from build123d import *

# Parameters (mm, degrees)
F0_R     = 20
F1_DEPTH = 20
F2_R     = 10
F3_R     = 9
F4_DEPTH = 20
F5_R     = 2.5
F6_DEPTH = 20
F7_SIZE  = 1.5


with BuildPart() as f1:
    # F0 (on Top) → F1 (new body)
    with BuildSketch(Plane.XY):
        Circle(F0_R)
    extrude(amount=F1_DEPTH)

    # F2
    f2_edges = [f1.edges().sort_by_distance(p)[0] for p in [
        (-20, 0, 0),
    ]]
    fillet(f2_edges, radius=F2_R)

    # F3 (on face) → F4 (join)
    with BuildSketch(Plane.XY.offset(20)):
        Circle(F3_R)
    extrude(amount=F4_DEPTH)

    # F5 (on face) → F6 (cut)
    with BuildSketch(Plane.XY.offset(40)):
        Circle(F5_R)
    extrude(amount=-F6_DEPTH, mode=Mode.SUBTRACT)

    # F7
    f7_edges = [f1.edges().sort_by_distance(p)[0] for p in [
        (-20, 0, 20),
    ]]
    chamfer(f7_edges, length=F7_SIZE)


solid = f1.part
Could you check a few things on this model? Use its own coordinates, in mm. A direction names the side the tool comes from. Coordinates: 2 decimals unless noted, no trailing zeros. Order: outer loops, then holes, each group sorted by start corner. A loop starts at its lowest first (then second) coordinate and runs counter-clockwise, first axis right, second up. Notation, with made-up numbers: (12, -27.75) - (62, -27.75) arc R11 cw to (62, -8.75) - close; hole circle Ø6 at (61.25, 8.25). An arc over 180 degrees is marked (long way). Answer in a Markdown table with one row per item. Add a question column.
(1) Will these pins go through, and if not, where does the flat tip stop? pin 1 (2 mm diameter, centred on x = 0, y = 15.5, fed in from +Z); pin 2 (1 mm diameter, centred on y = 0.5, z = 33, fed in from -X); pin 3 (1.5 mm diameter, centred on x = -3.5, z = 32.5, fed in from +Y).
(2) If we section it at A-A, the plane z = 34: Please give me the cut outline in (x, y), then the cut area to 3 significant figures.
(3) I need wall thicknesses on L1, parallel to Y at x = 0, z = 33.25; L2, parallel to Y at x = 7, z = 24.5; L3, parallel to Y at x = -17, z = 5. Which ranges of each line are inside material? Lowest first, please.
(4) On a 3-axis mill with a long thin cutter (end or side, diameter ignored), from which of +Z, -Z, +X, -X, +Y, -Y can I reach the whole of each face in a straight line? I mean faces 4 (the face through (2, -2, 40)), 5 (the face through (-0.54, -2.44, 30.14)). Say none if no direction works.
(5) If we mould it in two halves opening along Y, with no side actions, what happens to faces 1 (the face through (3.9, 8.5, 20)), 2 (the face through (0, 0, 20)), 3 (the face through (-4.336, -19.524, 14.19))? For each: released by +Y, released by -Y, zero draft, split by the parting line, or undercut.
Results are:
| question | item | result |
|---|---|---|
| 1 | pin 1 | stops at z = 20 |
| 1 | pin 2 | stops at x = -9 |
| 1 | pin 3 | stops at y = 8.57 |
| 2 | outline | circle Ø18 at (0, 0); hole circle Ø5 at (0, 0) |
| 2 | area | 235 mm2 |
| 3 | L1 | y = -9 to -2.5, 2.5 to 9 |
| 3 | L2 | y = -5.66 to 5.66 |
| 3 | L3 | y = -7.69 to 7.69 |
| 4 | face 4 | +Z, +X, -X, +Y, -Y |
| 4 | face 5 | +Z |
| 5 | face 1 | zero draft |
| 5 | face 2 | undercut |
| 5 | face 3 | split by the parting line |
